For this review, take the finished solid that the model builds, in its own axes (mm). Face numbers are marked on the shaded views. A direction names the side the tool comes from. Give positions to 0.01 mm unless a question says otherwise; leave off trailing zeros. Write each loop counter-clockwise with the first axis right and the second up, starting at its lowest first coordinate (ties: lowest second). Pieces come first, ordered by that corner, then holes. Notation, with made-up numbers: M 7.25,68.5 L 21.25,68.5 A14 ccw 21.25,94.5 Z; hole C 61.25,22 d8. An arc over 180 degrees is marked long. Write item = value, one per line.
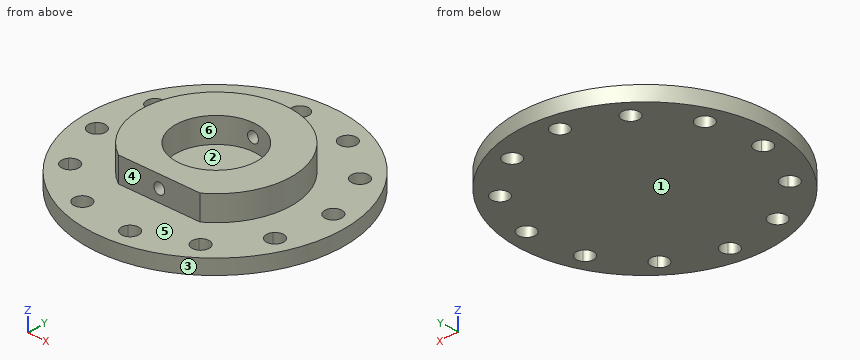
```python
from build123d import *

# Parameters (mm, degrees)
SKETCH1_R           = 25.608746635
BOSS_EXTRUDE1_DEPTH = 3
SKETCH2_R           = 8.1
BOSS_EXTRUDE2_DEPTH = 5


with BuildPart() as part:
    # Sketch1 → Boss-Extrude1 (new body)
    with BuildSketch(Plane.XY):
        with Locations((-0.244898521, 0)):
            Circle(SKETCH1_R)
        with BuildLine():
            ThreePointArc((-18.841121629, 7.385104949), (-19.140852563, 9.804238645), (-21.559986259, 9.504507711))
            ThreePointArc((-21.559986259, 9.504507711), (-21.260255325, 7.085374015), (-18.841121629, 7.385104949))
        make_face(mode=Mode.SUBTRACT)
        with BuildLine():
            ThreePointArc((-20.389973917, -3.72411228), (-20.689704851, -1.304978585), (-23.108838546, -1.604709519))
            ThreePointArc((-23.108838546, -1.604709519), (-22.809107612, -4.023843215), (-20.389973917, -3.72411228))
        make_face(mode=Mode.SUBTRACT)
        with BuildLine():
            ThreePointArc((-16.176710729, -14.119402761), (-16.476441664, -11.700269066), (-18.895575359, -12))
            ThreePointArc((-18.895575359, -12), (-18.595844425, -14.419133695), (-16.176710729, -14.119402761))
        make_face(mode=Mode.SUBTRACT)
        with BuildLine():
            ThreePointArc((-7.330272536, -21.015356804), (-7.63000347, -18.596223108), (-10.049137166, -18.895954043))
            ThreePointArc((-10.049137166, -18.895954043), (-9.749406231, -21.315087738), (-7.330272536, -21.015356804))
        make_face(mode=Mode.SUBTRACT)
        with BuildLine():
            ThreePointArc((3.778944694, -22.564209091), (3.479213759, -20.145075396), (1.060080064, -20.44480633))
            ThreePointArc((1.060080064, -20.44480633), (1.359810998, -22.863940025), (3.778944694, -22.564209091))
        make_face(mode=Mode.SUBTRACT)
        with BuildLine():
            ThreePointArc((11.455370545, -16.231543143), (11.755101479, -18.650676838), (14.174235175, -18.350945904))
            ThreePointArc((14.174235175, -18.350945904), (13.87450424, -15.931812209), (11.455370545, -16.231543143))
        make_face(mode=Mode.SUBTRACT)
        with BuildLine():
            ThreePointArc((18.351324588, -7.385104949), (18.651055522, -9.804238645), (21.070189217, -9.504507711))
            ThreePointArc((21.070189217, -9.504507711), (20.770458283, -7.085374015), (18.351324588, -7.385104949))
        make_face(mode=Mode.SUBTRACT)
        with BuildLine():
            ThreePointArc((22.619041505, 1.604709519), (22.31931057, 4.023843215), (19.900176875, 3.72411228))
            ThreePointArc((19.900176875, 3.72411228), (20.199907809, 1.304978585), (22.619041505, 1.604709519))
        make_face(mode=Mode.SUBTRACT)
        with BuildLine():
            ThreePointArc((15.686913688, 14.119402761), (15.986644622, 11.700269066), (18.405778317, 12))
            ThreePointArc((18.405778317, 12), (18.106047383, 14.419133695), (15.686913688, 14.119402761))
        make_face(mode=Mode.SUBTRACT)
        with BuildLine():
            ThreePointArc((6.840475494, 21.015356804), (7.140206429, 18.596223108), (9.559340124, 18.895954043))
            ThreePointArc((9.559340124, 18.895954043), (9.25960919, 21.315087738), (6.840475494, 21.015356804))
        make_face(mode=Mode.SUBTRACT)
        with BuildLine():
            ThreePointArc((-4.268741735, 22.564209091), (-3.969010801, 20.145075396), (-1.549877106, 20.44480633))
            ThreePointArc((-1.549877106, 20.44480633), (-1.84960804, 22.863940025), (-4.268741735, 22.564209091))
        make_face(mode=Mode.SUBTRACT)
        with BuildLine():
            ThreePointArc((-14.664032216, 18.350945904), (-14.364301282, 15.931812209), (-11.945167587, 16.231543143))
            ThreePointArc((-11.945167587, 16.231543143), (-12.244898521, 18.650676838), (-14.664032216, 18.350945904))
        make_face(mode=Mode.SUBTRACT)
    extrude(amount=BOSS_EXTRUDE1_DEPTH)

    # Sketch2 → Boss-Extrude2 (add)
    with BuildSketch(Plane.XY.offset(3)):
        with BuildLine():
            Line((8.291561976, -12.5), (-8.291561976, -12.5))
            ThreePointArc((-8.291561976, -12.5), (0, 15), (8.291561976, -12.5))
        make_face()
        Circle(SKETCH2_R, mode=Mode.SUBTRACT)
    extrude(amount=BOSS_EXTRUDE2_DEPTH)

    # Sketch4 → CBORE for M2 SHCS1 (revolve, cut)
    with BuildSketch(Plane(origin=(0, 15, 5.5), x_dir=(0, 0, 1), z_dir=(1, 0, 0))):
        Polygon((0, 0), (0, 40.608746635), (1.1, 40.608746635), (1.1, 2), (2.2, 2), (2.2, 0.025), (2.225, 0), align=None)
    revolve(axis=Axis((0, 21.35, 5.5), (0, -1, 0)), mode=Mode.SUBTRACT)


solid = part.part
```
1. The part is to be moulded in two halves that separate along Y. For the marked faces 3, 4, 5 and 6, say which applies: +Y half, -Y half, draft (parallel to the pull), parting line (faces both ways), or undercut.
Responses:
face_3 = parting line
face_4 = -Y half
face_5 = draft
face_6 = undercut
2. For line 1 along Y through (x, z) = (1, 6.5); line 2 along Y through (x, z) = (-19, 1); line 3 along X through (y, z) = (17, 2), list the stretches that pass through material, from the lowest coordinate up. Write a range as from..to.
Responses:
line_1 = -12.5..-8.04, 8.04..13
line_2 = -17.44..-13.97, -12.15..7.21, 9.68..17.44
line_3 = -19.4..-15, -11.61..18.91
3. We need section B-B, the plane x = 16.5. Write out the cut boundary in (y, z).
Responses:
outline = M -19.38,0 L 11.42,0 L 11.42,3 L -19.38,3 Z; M 14.69,0 L 19.38,0 L 19.38,3 L 14.69,3 Z
4. Insertion check: P1, Ø3, axis at y = 12.5, z = 1.5, coming from the +X side; P2, Ø14.5, axis at x = 0, y = 0, coming from the +Z side; P3, Ø3, axis at x = -11, z = 2.5, coming from the +Y side. Each pin has a flat end and moves straight along its axis. Give the tip position at first contact, or say it passes through.
Responses:
P1 = 22.88
P2 = 3
P3 = 23.88
5. Machinability: for the marked faces 1 and 2, which of the approach directions +Z, -Z, +X, -X, +Y, -Y give a long, thin tool a straight path to every point of the face, cutting with its end or side? Answer none if there is none.
Responses:
face_1 = -Z, +X, -X, +Y, -Y
face_2 = +Z
6. We need section D-D, the plane y = 5. Write out the cut boundary in (x, z), then the cut area to 3 significant figures.
Responses:
outline = M -25.36,0 L 24.87,0 L 24.87,3 L 14.14,3 L 14.14,8 L 6.37,8 L 6.37,3 L -6.37,3 L -6.37,8 L -14.14,8 L -14.14,3 L -25.36,3 Z
area = 228 mm2
7. We need section C-C, the plane x = 0. Write out the cut boundary in (y, z) (3 decimals).
Responses:
outline = M -25.608,0 L 25.608,0 L 25.608,3 L 15,3 L 15,3.275 L 14.975,3.3 L 13,3.3 L 13,4.4 L 8.1,4.4 L 8.1,3 L -8.1,3 L -8.1,4.4 L -12.5,4.4 L -12.5,3 L -25.608,3 Z; M -12.5,6.6 L -8.1,6.6 L -8.1,8 L -12.5,8 Z; M 8.1,6.6 L 13,6.6 L 13,7.7 L 14.975,7.7 L 15,7.725 L 15,8 L 8.1,8 Z
8. We need section A-A, the plane z = 5.25. Write out the cut boundary in (x, y), then the cut area to 3 significant figures.
Responses:
outline = M -8.29,-12.5 L -1.07,-12.5 L -1.07,-8.03 A8.1 cw -1.07,8.03 L -1.07,13 L -2.19,13 L -2.19,14.84 A15 ccw Z; M 1.07,-12.5 L 8.29,-12.5 A15 ccw 2.19,14.84 L 2.19,13 L 1.07,13 L 1.07,8.03 A8.1 cw 1.07,-8.03 Z
area = 444 mm2
